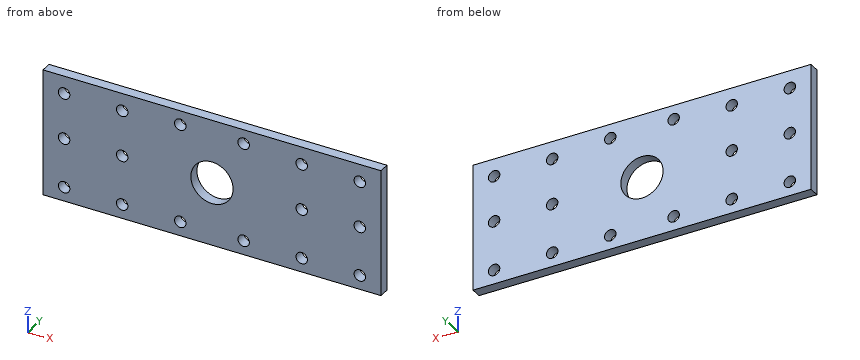
from build123d import *

# Parameters (mm, degrees)
F0_R     = 10.31875
F0_R_2   = 38.1
F1_DEPTH = 19.05


with BuildPart() as f1:
    # F0 (on Front) → F1 (new body)
    with BuildSketch(Plane.XZ):
        with BuildLine():
            ThreePointArc((31.590851, 85.725), (0, -19.05), (-31.590851, 85.725))
            Line((-31.590851, 85.725), (-304.8, 85.725))
            Line((-304.8, 85.725), (-304.8, -76.2))
            Line((-304.8, -76.2), (295.275, -76.2))
            Line((295.275, -76.2), (295.275, 76.2))
            ThreePointArc((295.275, 76.2), (292.485192, 82.935192), (285.75, 85.725))
            Line((285.75, 85.725), (31.590851, 85.725))
        make_face()
        with Locations((-266.7, -50.8)):
            Circle(F0_R, mode=Mode.SUBTRACT)
        with Locations((-161.925, -50.8)):
            Circle(F0_R, mode=Mode.SUBTRACT)
        with Locations((-57.15, -50.8)):
            Circle(F0_R, mode=Mode.SUBTRACT)
        with Locations((57.15, -50.8)):
            Circle(F0_R, mode=Mode.SUBTRACT)
        with Locations((161.925, -50.8)):
            Circle(F0_R, mode=Mode.SUBTRACT)
        with Locations((-266.7, 38.1)):
            Circle(F0_R, mode=Mode.SUBTRACT)
        with Locations((-161.925, 38.1)):
            Circle(F0_R, mode=Mode.SUBTRACT)
        with Locations((161.925, 38.1)):
            Circle(F0_R, mode=Mode.SUBTRACT)
        with Locations((266.7, -50.8)):
            Circle(F0_R, mode=Mode.SUBTRACT)
        with Locations((266.7, 38.1)):
            Circle(F0_R, mode=Mode.SUBTRACT)
        with BuildLine():
            Line((0, 85.725), (-31.590851, 85.725))
            ThreePointArc((-31.590851, 85.725), (0, -19.05), (31.590851, 85.725))
            Line((31.590851, 85.725), (0, 85.725))
        make_face()
        with Locations((0, 38.1)):
            Circle(F0_R_2, mode=Mode.SUBTRACT)
        Polygon((-304.8, 152.4), (-304.8, 95.25), (0, 95.25), (304.8, 95.25), (304.8, 152.4), align=None)
        with Locations((-266.7, 120.65)):
            Circle(F0_R, mode=Mode.SUBTRACT)
        with Locations((-161.925, 120.65)):
            Circle(F0_R, mode=Mode.SUBTRACT)
        with Locations((-57.15, 127)):
            Circle(F0_R, mode=Mode.SUBTRACT)
        with Locations((57.15, 127)):
            Circle(F0_R, mode=Mode.SUBTRACT)
        with Locations((161.925, 120.65)):
            Circle(F0_R, mode=Mode.SUBTRACT)
        with Locations((266.7, 120.65)):
            Circle(F0_R, mode=Mode.SUBTRACT)
        Polygon((-304.8, 85.725), (-31.590851, 85.725), (0, 85.725), (31.590851, 85.725), (285.75, 85.725), (304.8, 85.725), (304.8, 95.25), (0, 95.25), (-304.8, 95.25), align=None)
        with BuildLine():
            Line((304.8, 85.725), (285.75, 85.725))
            ThreePointArc((285.75, 85.725), (292.485192, 82.935192), (295.275, 76.2))
            Line((295.275, 76.2), (295.275, -76.2))
            Line((295.275, -76.2), (304.8, -76.2))
            Line((304.8, -76.2), (304.8, 47.625))
            Line((304.8, 47.625), (304.8, 85.725))
        make_face()
    extrude(amount=-F1_DEPTH)


solid = f1.part
Source: CAD feature listing. Evaluate the final solid. Frame: model axes, mm. Give positions to 0.01 mm unless a question says otherwise; leave off trailing zeros. Write each loop counter-clockwise with the first axis right and the second up, starting at its lowest first coordinate (ties: lowest second). Pieces come first, ordered by that corner, then holes. Notation, with made-up numbers: M -39,-24 L -19,-24 A22 cw -19,-10 Z; hole C 70,72 d8. An arc over 180 degrees is marked long. Return JSON: item names as keys, results as strings. Group by question number.
1) Cut plane C-C, the plane z = 38.1. Output: boundary loops of the cut face in (x, y).
2) Ray query, L1, parallel to Z at x = 57.15, y = 14.75; L2, parallel to Z at x = 167.5, y = 11.5; L3, parallel to Z at x = 258, y = 4.25. Return the intervals inside material, ascending.
3) Cut plane B-B, the plane x = 266.7. Output: boundary loops of the cut face in (y, z), then the cut area to 3 significant figures.
4) Cut plane A-A, the plane z = -50.8. Output: boundary loops of the cut face in (x, y).
5) Cut plane D-D, the plane x = 0. Output: boundary loops of the cut face in (y, z), then the cut area to 3 significant figures.
6) First-contact query: pin 1 Ø18.5 at (x, z) = (-266.7, 120.65) entering from +Y (1 decimal). Flat tip, straight axial feed; report the tip coordinate or a pass-through.
Data:
{
 "1": {"outline": "M -304.8,0 L -277.02,0 L -277.02,19.05 L -304.8,19.05 Z; M -256.38,0 L -172.24,0 L -172.24,19.05 L -256.38,19.05 Z; M -151.61,0 L -38.1,0 L -38.1,19.05 L -151.61,19.05 Z; M 38.1,0 L 151.61,0 L 151.61,19.05 L 38.1,19.05 Z; M 172.24,0 L 256.38,0 L 256.38,19.05 L 172.24,19.05 Z; M 277.02,0 L 304.8,0 L 304.8,19.05 L 277.02,19.05 Z"},
 "2": {"L1": "z = -76.2 to -61.12, -40.48 to 116.68, 137.32 to 152.4", "L2": "z = -76.2 to -59.48, -42.12 to 29.42, 46.78 to 111.97, 129.33 to 152.4", "L3": "z = -76.2 to -56.35, -45.25 to 32.55, 43.65 to 115.1, 126.2 to 152.4"},
 "3": {"outline": "M 0,-76.2 L 19.05,-76.2 L 19.05,-61.12 L 0,-61.12 Z; M 0,-40.48 L 19.05,-40.48 L 19.05,27.78 L 0,27.78 Z; M 0,48.42 L 19.05,48.42 L 19.05,110.33 L 0,110.33 Z; M 0,130.97 L 19.05,130.97 L 19.05,152.4 L 0,152.4 Z", "area": "3,180 mm²"},
 "4": {"outline": "M -304.8,0 L -277.02,0 L -277.02,19.05 L -304.8,19.05 Z; M -256.38,0 L -172.24,0 L -172.24,19.05 L -256.38,19.05 Z; M -151.61,0 L -67.47,0 L -67.47,19.05 L -151.61,19.05 Z; M -46.83,0 L 46.83,0 L 46.83,19.05 L -46.83,19.05 Z; M 67.47,0 L 151.61,0 L 151.61,19.05 L 67.47,19.05 Z; M 172.24,0 L 256.38,0 L 256.38,19.05 L 172.24,19.05 Z; M 277.02,0 L 304.8,0 L 304.8,19.05 L 277.02,19.05 Z"},
 "5": {"outline": "M 0,-76.2 L 19.05,-76.2 L 19.05,0 L 0,0 Z; M 0,76.2 L 19.05,76.2 L 19.05,152.4 L 0,152.4 Z", "area": "2,900 mm²"},
 "6": {"pin 1": "passes through"}
}
